Geometry: see drawing. Coordinates: mm, zero at the bounding-box minimum. Coordinates: 2 decimals unless noted, no trailing zeros. Write each loop counter-clockwise with the first axis right and the second up, starting at its lowest first coordinate (ties: lowest second). Pieces come first, ordered by that corner, then holes. Notation, with made-up numbers: M -35,8 L 13,8 A34 cw 13,42 Z; hole C 45,23 d7. An arc over 180 degrees is marked long. Write item = value, one per line. Start each with the question number.
1. Section query C-C (y = 22). Output: boundary loops of the cut face in (x, z).
2. Pin query (flat end, axial travel): pin 1 Ø4.5 at (x, y) = (2.7, 33.7) entering from +Z; pin 2 Ø3 at (x, y) = (2.7, 2.7) entering from +Z; pin 3 Ø3 at (y, z) = (13, 7.5) entering from -X; pin 4 Ø1.9 at (x, z) = (45, 6.5) entering from -Y. Return the tip coordinate at first contact, or that it passes through.
3. Section query A-A (y = 33.7). Output: boundary loops of the cut face in (x, z), then the cut area to 3 significant figures.
4. Section query B-B (x = 77.7). Output: boundary loops of the cut face in (y, z), then the cut area to 3 significant figures.
5. Section query D-D (x = 15). Output: boundary loops of the cut face in (y, z), then the cut area to 3 significant figures.
6. Line query: line 1 along X through (y, z) = (2.7, 1.6); line 2 along Y through (x, z) = (77.7, 2.2); line 3 along X through (y, z) = (7, 8.25). Output: solid intervals per line, ascending.
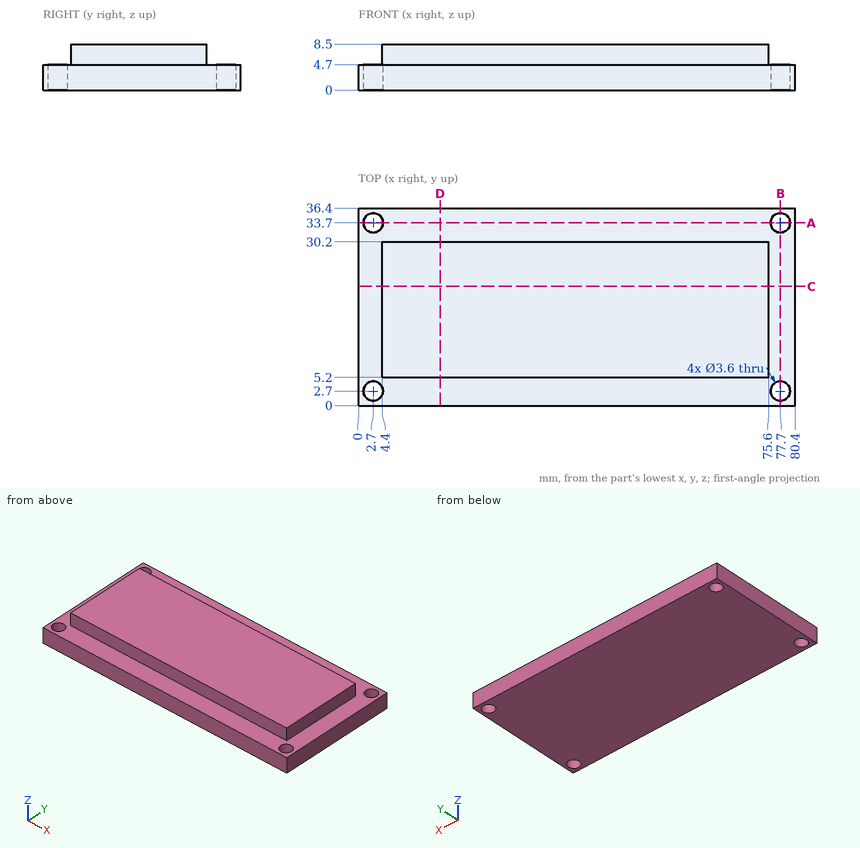
Results are:
q1.outline = M 0,0 L 80.4,0 L 80.4,4.7 L 75.6,4.7 L 75.6,8.5 L 4.4,8.5 L 4.4,4.7 L 0,4.7 Z
q2.pin_1 = 4.7
q2.pin_2 = through
q2.pin_3 = 4.4
q2.pin_4 = 5.2
q3.outline = M 0,0 L 0.9,0 L 0.9,4.7 L 0,4.7 Z; M 4.5,0 L 75.9,0 L 75.9,4.7 L 4.5,4.7 Z; M 79.5,0 L 80.4,0 L 80.4,4.7 L 79.5,4.7 Z
q3.area = 344 mm^2
q4.outline = M 0,0 L 0.9,0 L 0.9,4.7 L 0,4.7 Z; M 4.5,0 L 31.9,0 L 31.9,4.7 L 4.5,4.7 Z; M 35.5,0 L 36.4,0 L 36.4,4.7 L 35.5,4.7 Z
q4.area = 137 mm^2
q5.outline = M 0,0 L 36.4,0 L 36.4,4.7 L 30.2,4.7 L 30.2,8.5 L 5.2,8.5 L 5.2,4.7 L 0,4.7 Z
q5.area = 266 mm^2
q6.line_1 = 0 to 0.9, 4.5 to 75.9, 79.5 to 80.4
q6.line_2 = 0 to 0.9, 4.5 to 31.9, 35.5 to 36.4
q6.line_3 = 4.4 to 75.6
